Autodesk Inventor part; units mm, degrees
ref_plane "YZ Plane" through (0, 0, 0) normal (1, 0, 0) x (0, 1, 0)
ref_plane "XZ Plane" through (0, 0, 0) normal (0, 1, 0) x (-1, 0, 0)
ref_plane "XY Plane" through (0, 0, 0) normal (0, 0, 1) x (1, 0, 0)
sketch "스케치4" plane through (0, 0, 0) normal (0, 1, 0) x (-1, 0, 0)
  line L0 (-2, 5.5) -> (-2, -5.5)
  line L1 (-2, -5.5) -> (2, -5.5)
  line L2 (2, -5.5) -> (2, 5.5)
  line L3 (2, 5.5) -> (-2, 5.5)
  line L4 (-2, 5.5) -> (2, -5.5) construction
  line L5 (-2, -5.5) -> (2, 5.5) construction
  point P0 (0, 0)
  point P1 (0, 0)
  dimension "d12" = 11
  dimension "d13" = 4
extrude "돌출3" add sketch "스케치4" along normal blind 77
sketch "스케치5" plane through (0, 0, 0) normal (0, -1, 0) x (1, 0, 0)
  line L0 (-10.5, -5.5) -> (10.5, -5.5)
  line L1 (10.5, -5.5) -> (10.5, 5.5)
  line L2 (10.5, 5.5) -> (-10.5, 5.5)
  line L3 (-10.5, 5.5) -> (-10.5, -5.5)
  line L4 (-10.5, -5.5) -> (10.5, 5.5) construction
  line L5 (10.5, -5.5) -> (-10.5, 5.5) construction
  line L6 (0, 5.5) -> (0, -5.5) construction
  line L7 (10.5, 5.5) -> (12.5, 5.5)
  line L8 (12.5, 5.5) -> (12.5, -5.5)
  line L9 (12.5, -5.5) -> (10.5, -5.5)
  line L10 (-10.5, 5.5) -> (-12.5, 5.5)
  line L11 (-12.5, 5.5) -> (-12.5, -5.5)
  line L12 (-12.5, -5.5) -> (-10.5, -5.5)
  line L13 (-22.4262, 19.8) -> (40.7349, 19.8) construction
  point P0 (0, 0)
  point P1 (0, 0)
  dimension "d16" = 21
  dimension "d17" = 11
  dimension "d18" = 2
  dimension "d43" = 19.8
extrude "돌출4" add sketch "스케치5" along normal blind 2
extrude "돌출5" add sketch "스케치5" along normal blind 22 contours L12 L11 L10 L3 | L1 L7 L8 L9
sketch "스케치6" plane through (-12.5, 0, -5.5) normal (-1, 0, 0) x (0, 0, 1)
  line L0 (11, 0) -> (0, 0)
  line L1 (0, 0) -> (0, -22)
  line L2 (11, -22) -> (0, -22)
  line L3 (11, 0) -> (11, -22)
  circle A0 centre (5.5, -12) radius 1.5
  point P0 (5.5, 0)
  dimension "d23" = 3
  dimension "d24" = 10
extrude "돌출6" cut sketch "스케치6" against normal through all contours A0
sketch "스케치7" plane through (-2, 77, -5.5) normal (-1, 0, 0) x (0, 0, 1)
  line L0 (0, -77) -> (11, -77)
  line L1 (11, -77) -> (11, 0)
  line L2 (0, 0) -> (11, 0)
  line L3 (0, -77) -> (0, 0)
  line L4 (0, -73) -> (11, -73) construction
  line L5 (0, -4) -> (11, -4) construction
  line L6 (0, -69) -> (11, -69) construction
  circle A0 centre (5.5, -4) radius 1.5
  circle A1 centre (5.5, -69) radius 1.5
  line L7 (5.5, -69) -> (5.5, -4) construction
  circle A2 centre (5.5, -64) radius 1.5
  circle A3 centre (5.5, -59) radius 1.5
  circle A4 centre (5.5, -54) radius 1.5
  circle A5 centre (5.5, -49) radius 1.5
  circle A6 centre (5.5, -44) radius 1.5
  circle A7 centre (5.5, -39) radius 1.5
  circle A8 centre (5.5, -34) radius 1.5
  circle A9 centre (5.5, -29) radius 1.5
  circle A10 centre (5.5, -24) radius 1.5
  circle A11 centre (5.5, -19) radius 1.5
  circle A12 centre (5.5, -14) radius 1.5
  circle A13 centre (5.5, -9) radius 1.5
  point P0 (5.5, -77)
  dimension "d27" = 4
  dimension "d28" = 4
  dimension "d29" = 4
  dimension "d30" = 3
  dimension "d31" = 5.5
  dimension "d32" = 3
  dimension "d35" = 5
extrude "돌출7" cut sketch "스케치7" against normal through all contours A0 | A1 | A2 | A3 | A4 | A5 | A6 | A7 | A8 | A9 | A10 | A11 | A12 | A13
properties part number "catcher"
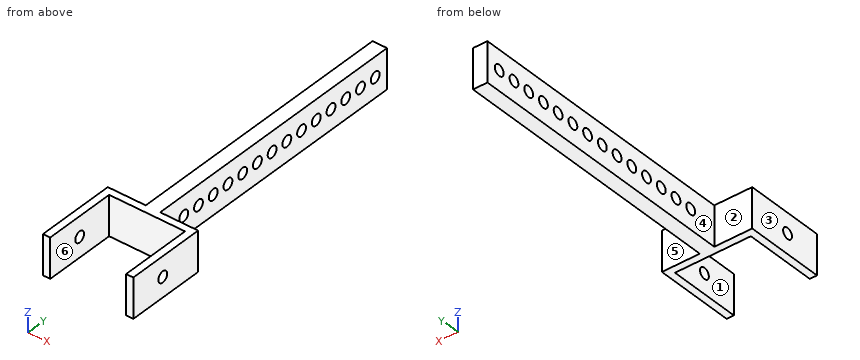
Read the model definition and answer for the solid it produces. Units are mm, in the model's axes. Face numbers are marked on the shaded views. A direction names the side the tool comes from. Coordinates: 2 decimals unless noted, no trailing zeros. Order: outer loops, then holes, each group sorted by start corner. A loop starts at its lowest first (then second) coordinate and runs counter-clockwise, first axis right, second up. Notation, with made-up numbers: (45.5, 33) - (60.5, 33) arc R18 cw to (60.5, 61) - close; hole circle Ø8 at (50, 2). An arc over 180 degrees is marked (long way). Answer as a JSON object with one key per item and string values. Group by question number.
Item 1: Flat-ended cylindrical pins translate along their axes: P1, Ø5.5, axis at y = 40, z = 1, coming from the +X side; P2, Ø3, axis at y = 54, z = -1.5, coming from the -X side; P3, Ø2.5, axis at y = 63, z = 0, coming from the +X side; P4, Ø5.5, axis at x = -2.5, z = -2, coming from the -Y side. Find the tip coordinate at first contact, or state that the pin passes through.
Item 2: A tool of negligible diameter and unlimited length cuts with its end or side. For the marked faces 1, 2 and 3, from which of +Z, -Z, +X, -X, +Y, -Y can it reach the whole face along a straight path? Write none if from no direction.
Item 3: Section B-B (x = 1) is taken. State how many separate pieces and enclosed holes the cut face has, plus the area to 3 significant figures.
Item 4: Section C-C (z = 3.25) is taken. Give the vertices of the cut face in (x, y), plus the area to 3 significant figures.
Item 5: The mould has two halves that part along X. Classify the marked faces 4, 5 and 6: +X half, -X half, draft (parallel to the pull), parting line (faces both ways), or undercut.
Item 6: Section A-A (y = 8) is taken. Give the vertices of the cut face in (x, z), plus the area to 3 significant figures.
Item 7: Consider probe 1 along X at (y, z) = (-14, 3.5); probe 2 along X at (y, z) = (64.5, -4.75); probe 3 along Y at (x, z) = (-3.25, 4.25). Determine where each line is inside the solid, lowest interval first. Write a range as from..to.
Item 8: Section D-D (y = -6.5) is taken. Give the vertices of the cut face in (x, z).
Results are:
{
 "1": {"P1": "stops at x = 2", "P2": "stops at x = -2", "P3": "passes through", "P4": "stops at y = -2"},
 "2": {"face 1": "+Z, -Z, -Y", "face 2": "+Z, -Z, -X, +Y", "face 3": "+Z, -Z, -X, +Y, -Y"},
 "3": {"separate pieces": "1", "enclosed holes": "14", "area": "770 mm^2"},
 "4": {"outline": "(-12.5, -22) - (-10.5, -22) - (-10.5, -2) - (10.5, -2) - (10.5, -22) - (12.5, -22) - (12.5, 0) - (2, 0) - (2, 77) - (-2, 77) - (-2, 0) - (-12.5, 0) - close", "area": "438 mm^2"},
 "5": {"face 4": "-X half", "face 5": "draft", "face 6": "undercut"},
 "6": {"outline": "(-2, -5.5) - (2, -5.5) - (2, -1.5) - (-2, -1.5) - close; (-2, 1.5) - (2, 1.5) - (2, 5.5) - (-2, 5.5) - close", "area": "32.0 mm^2"},
 "7": {"probe 1": "x = -12.5..-10.5, 10.5..12.5", "probe 2": "x = -2..2", "probe 3": "y = -2..0"},
 "8": {"outline": "(-12.5, -5.5) - (-10.5, -5.5) - (-10.5, 5.5) - (-12.5, 5.5) - close; (10.5, -5.5) - (12.5, -5.5) - (12.5, 5.5) - (10.5, 5.5) - close"}
}
